Design review of the part built by this model. Coordinates are the model's own, in mm. Face numbers are marked on the shaded views. A direction names the side the tool comes from. Coordinates: 2 decimals unless noted, no trailing zeros. Write each loop counter-clockwise with the first axis right and the second up, starting at its lowest first coordinate (ties: lowest second). Pieces come first, ordered by that corner, then holes. Notation, with made-up numbers: (57.5, -27) - (101.5, -27) arc R27 cw to (101.5, 9) - close; hole circle Ø5 at (-18.5, -31.5). An arc over 180 degrees is marked (long way). Use a Markdown table: item, result.
from build123d import *

# Parameters (mm, degrees)
SKETCH_1_R               = 25
EXTRUDE_1_DEPTH          = 30
SKETCH_2_R               = 27.5
EXTRUDE_2_DEPTH          = 5
EXTRUDE_START            = 11
SKETCH_3_R               = 25
EXTRUDE_3_DEPTH          = 11
SKETCH_4_R               = 14
EXTRUDE_4_DEPTH          = 43
SKETCH_5_R               = 12.5
EXTRUDE_5_DEPTH          = 27
SKETCH_6_R               = 8.5
EXTRUDE_6_DEPTH          = 12
CUT_EXTRUDE_1_DEPTH      = 4
CUT_EXTRUDE_1_DEPTH_BACK = 4
SKETCH_7_W               = 4
SKETCH_7_H               = 30
FILLET_1_R               = 4
CHAMFER_1_SIZE           = 1
SKETCH_8_R               = 22.5
EXTRUDE_7_DEPTH          = 35
CHAMFER_2_SIZE           = 1
SKETCH_9_R               = 13
CUT_EXTRUDE_2_DEPTH      = 40
CHAMFER_3_SIZE           = 1
CUT_EXTRUDE_3_DEPTH      = 34


with BuildPart() as part:
    # 草图1 → 凸台-拉伸1 (new body)
    with BuildSketch(Plane.XY):
        Circle(SKETCH_1_R)
    extrude(amount=EXTRUDE_1_DEPTH)

    # 草图2 → 凸台-拉伸2 (add)
    with BuildSketch(Plane(origin=(0, 0, 0), x_dir=(-1, 0, 0), z_dir=(0, 0, -1))):
        Circle(SKETCH_2_R)
    extrude(amount=EXTRUDE_2_DEPTH)

    # 草图3 → 凸台-拉伸3 (add)
    with BuildSketch(Plane(origin=(0, 0, -5), x_dir=(-1, 0, 0), z_dir=(0, 0, -1)).offset(EXTRUDE_START)):
        Circle(SKETCH_3_R)
    extrude(amount=-EXTRUDE_3_DEPTH)

    # 草图4 → 凸台-拉伸4 (add)
    with BuildSketch(Plane(origin=(0, 0, -16), x_dir=(-1, 0, 0), z_dir=(0, 0, -1))):
        Circle(SKETCH_4_R)
    extrude(amount=EXTRUDE_4_DEPTH)

    # 草图5 → 凸台-拉伸5 (add)
    with BuildSketch(Plane(origin=(0, 0, -59), x_dir=(-1, 0, 0), z_dir=(0, 0, -1))):
        Circle(SKETCH_5_R)
    extrude(amount=EXTRUDE_5_DEPTH)

    # 草图6 → 凸台-拉伸6 (add)
    with BuildSketch(Plane(origin=(0, 0, -86), x_dir=(-1, 0, 0), z_dir=(0, 0, -1))):
        Circle(SKETCH_6_R)
    extrude(amount=EXTRUDE_6_DEPTH)

    # 草图7 → 切除-拉伸1 (cut, two sides: drawn at the far end of the back side and taken through both)
    with BuildSketch(Plane(origin=(0, 0, 0), x_dir=(1, 0, 0), z_dir=(0, 1, 0)).offset(-CUT_EXTRUDE_1_DEPTH_BACK)):
        with Locations((12, 37.5)):
            Rectangle(SKETCH_7_W, SKETCH_7_H)
    extrude(amount=CUT_EXTRUDE_1_DEPTH + CUT_EXTRUDE_1_DEPTH_BACK, mode=Mode.SUBTRACT)

    # 圆角1
    fillet_1_edges = [part.edges().sort_by_distance(p)[0] for p in [
        (11.708203932, 4, -22.5),
        (11.708203932, -4, -22.5),
        (11.708203932, -4, -52.5),
        (11.708203932, 4, -52.5),
    ]]
    fillet(fillet_1_edges, radius=FILLET_1_R - 0.0001)  # a hair under: the kernel refuses the full size

    # 倒角1
    chamfer_1_edges = [part.edges().sort_by_distance(p)[0] for p in [
        (14, 0, -59),
        (12.5, 0, -86),
        (8.5, 0, -98),
    ]]
    chamfer(chamfer_1_edges, length=CHAMFER_1_SIZE)

    # 草图8 → 凸台-拉伸7 (add)
    with BuildSketch(Plane.XY.offset(30)):
        Circle(SKETCH_8_R)
    extrude(amount=EXTRUDE_7_DEPTH)

    # 倒角2
    chamfer_2_edges = [part.edges().sort_by_distance(p)[0] for p in [
        (-22.5, 0, 65),
    ]]
    chamfer(chamfer_2_edges, length=CHAMFER_2_SIZE)

    # 草图9 → 切除-拉伸2 (cut)
    with BuildSketch(Plane.XY.offset(65)):
        Circle(SKETCH_9_R)
    extrude(amount=-CUT_EXTRUDE_2_DEPTH, mode=Mode.SUBTRACT)

    # 倒角3
    chamfer_3_edges = [part.edges().sort_by_distance(p)[0] for p in [
        (-13, 0, 65),
    ]]
    chamfer(chamfer_3_edges, length=CHAMFER_3_SIZE)

    # 草图10 → 切除-拉伸3 (cut)
    with BuildSketch(Plane.XY.offset(65)):
        Polygon((-4, -13), (-4, -8.881570562), (4, -8.881570562), (4, -13), (4, -15.3), (-4, -15.3), align=None)
    extrude(amount=-CUT_EXTRUDE_3_DEPTH, mode=Mode.SUBTRACT)


solid = part.part
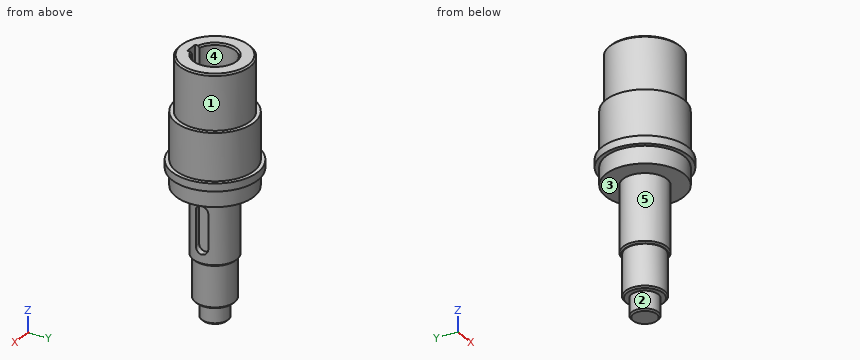
(1) Take a section at B-B on z = -33. Write out the cut boundary in (x, y), and give its area (3 significant figures).
Determined:
| item | result |
|---|---|
| outline | (10, -4) - (10, 4) - (13.42, 4) arc R14 ccw (long way) to (13.42, -4) - close |
| area | 585 mm2 |
(2) For L1, parallel to Y at x = 0, z = 49; L2, parallel to Z at x = -5, y = -24; L3, parallel to Y at x = -10.5, z = 41, list the stretches that pass through material, from the lowest coordinate up. Write a range as from..to.
Determined:
| item | result |
|---|---|
| L1 | -22.5..-15.3, 13..22.5 |
| L2 | -16..30 |
| L3 | -19.9..-7.66, 7.66..19.9 |
(3) Draft analysis for pull direction Y (two halves, no side actions). For the marked faces 3, 4 and 5, state which applies: +Y half, -Y half, draft (parallel to the pull), parting line (faces both ways), or undercut.
Determined:
| item | result |
|---|---|
| face 3 | draft |
| face 4 | undercut |
| face 5 | parting line |
(4) For pin 1 (5 mm diameter, centred on x = -18.5, y = -6, fed in from -Z); pin 2 (0.9 mm diameter, centred on y = -13.5, z = 54, fed in from +X); pin 3 (0.9 mm diameter, centred on x = 1.5, y = -14.5, fed in from +Z); pin 4 (1 mm diameter, centred on x = 5, y = -6, fed in from -Z), all flat-tipped, find the tip position at first contact; note any pin that passes through.
Determined:
| item | result |
|---|---|
| pin 1 | z = -16 |
| pin 2 | x = 18.33 |
| pin 3 | z = 31 |
| pin 4 | z = -98 |
(5) Take a section at D-D on z = -83. Write out the cut boundary in (x, y).
Determined:
| item | result |
|---|---|
| outline | circle Ø25 at (0, 0) |
(6) Machinability: for the marked faces 1 and 2, which of the approach directions +Z, -Z, +X, -X, +Y, -Y give a long, thin tool a straight path to every point of the face, cutting with its end or side? Answer none if there is none.
Determined:
| item | result |
|---|---|
| face 1 | +Z |
| face 2 | -Z |
(7) Take a section at A-A on z = 37. Write out the cut boundary in (x, y), and give its area (3 significant figures).
Determined:
| item | result |
|---|---|
| outline | circle Ø45 at (0, 0); hole (-4, -15.3) - (4, -15.3) - (4, -12.37) arc R13 ccw (long way) to (-4, -12.37) - close |
| area | 1,040 mm2 |
(8) Take a section at C-C on z = 6. Write out the cut boundary in (x, y).
Determined:
| item | result |
|---|---|
| outline | circle Ø50 at (0, 0) |
